Part model, mm, in its own coordinate system. A direction names the side the tool comes from. Coordinates: 2 decimals unless noted, no trailing zeros. Order: outer loops, then holes, each group sorted by start corner. A loop starts at its lowest first (then second) coordinate and runs counter-clockwise, first axis right, second up. Notation, with made-up numbers: M -12,-24.5 L 44,-24.5 A11 cw 44,-15.5 Z; hole C -37,83 d3. An arc over 180 degrees is marked long. Answer in a Markdown table with one row per item. Add a question column.
from build123d import *

# Parameters (mm, degrees)
SKETCH1_W             = 42
SKETCH1_H             = 42
BOSS_EXTRUDE1_DEPTH   = 36
SKETCH2_OUTSIDE_W     = 57.892
SKETCH2_OUTSIDE_H     = 57.892
SKETCH2_OUTSIDE_R     = 11
CUT_EXTRUDE1_DEPTH    = 2
FILLET1_R             = 0.5
SKETCH3_R             = 4
CUT_EXTRUDE2_DEPTH    = 3
SKETCH4_R             = 2.5
BOSS_EXTRUDE2_DEPTH   = 27
FILLET3_R             = 1
SKETCH5_R             = 12
BOSS_EXTRUDE3_DEPTH   = 0.5
FILLET4_R             = 0.1
M3_TAPPED_HOLE1_D     = 2.5
M3_TAPPED_HOLE1_DEPTH = 1
M3_TAPPED_HOLE1_TIP   = 0.751075774
CHAMFER2_SIZE         = 5
BOSS_EXTRUDE4_DEPTH   = 0.2
CUT_EXTRUDE4_START    = -10
CUT_EXTRUDE4_DEPTH    = 10
BOSS_EXTRUDE5_START   = -34.2
BOSS_EXTRUDE5_DEPTH   = 8
M3_TAPPED_HOLE3_D     = 2.5
M3_TAPPED_HOLE3_DEPTH = 1
M3_TAPPED_HOLE3_TIP   = 0.751075774


with BuildPart() as part:
    # Sketch1 → Boss-Extrude1 (new body)
    with BuildSketch(Plane.XY):
        Rectangle(SKETCH1_W, SKETCH1_H)
    extrude(amount=BOSS_EXTRUDE1_DEPTH)

    # Sketch2 outside → Cut-Extrude1 (cut)
    with BuildSketch(Plane.XY.offset(36)):
        Rectangle(SKETCH2_OUTSIDE_W, SKETCH2_OUTSIDE_H)
        Circle(SKETCH2_OUTSIDE_R, mode=Mode.SUBTRACT)
    extrude(amount=-CUT_EXTRUDE1_DEPTH, mode=Mode.SUBTRACT)

    # Fillet1
    fillet1_edges = [part.edges().sort_by_distance(p)[0] for p in [
        (-11, 0, 36),
    ]]
    fillet(fillet1_edges, radius=FILLET1_R)

    # Sketch3 → Cut-Extrude2 (cut)
    with BuildSketch(Plane.XY.offset(36)):
        Circle(SKETCH3_R)
    extrude(amount=-CUT_EXTRUDE2_DEPTH, mode=Mode.SUBTRACT)

    # Sketch4 → Boss-Extrude2 (add)
    with BuildSketch(Plane.XY.offset(33)):
        Circle(SKETCH4_R)
    extrude(amount=BOSS_EXTRUDE2_DEPTH)

    # Fillet3
    fillet3_edges = [part.edges().sort_by_distance(p)[0] for p in [
        (-2.5, 0, 60),
    ]]
    fillet(fillet3_edges, radius=FILLET3_R)

    # Sketch5 → Boss-Extrude3 (add)
    with BuildSketch(Plane.XY.offset(34)):
        Circle(SKETCH5_R)
    extrude(amount=BOSS_EXTRUDE3_DEPTH)

    # Fillet4
    fillet4_edges = [part.edges().sort_by_distance(p)[0] for p in [
        (-11, 0, 34.5),
    ]]
    fillet(fillet4_edges, radius=FILLET4_R)

    # M3 Tapped Hole1
    with Locations(Plane.XY.offset(34)):
        with Locations((15.5, 15.5), (-15.5, 15.5), (15.5, -15.5), (-15.5, -15.5)):
            Hole(M3_TAPPED_HOLE1_D / 2, depth=M3_TAPPED_HOLE1_DEPTH)
            with Locations((0, 0, -(M3_TAPPED_HOLE1_DEPTH + M3_TAPPED_HOLE1_TIP / 2))):  # 118° drill point
                Cone(0, M3_TAPPED_HOLE1_D / 2, M3_TAPPED_HOLE1_TIP, mode=Mode.SUBTRACT)

    # Chamfer2
    chamfer2_edges = [part.edges().sort_by_distance(p)[0] for p in [
        (21, -21, 17),
        (-21, -21, 17),
        (-21, 21, 17),
        (21, 21, 17),
    ]]
    chamfer(chamfer2_edges, length=CHAMFER2_SIZE)

    # Sketch9 → Boss-Extrude4 (add)
    with BuildSketch(Plane.XY.offset(34)):
        with BuildLine():
            Line((16, 21), (21, 16))
            Line((21, 16), (21, 10.138100447))
            Line((21, 10.138100447), (14.858342654, 10.138100447))
            ThreePointArc((14.858342654, 10.138100447), (11.322808748, 11.602566541), (9.858342654, 15.138100447))
            Line((9.858342654, 15.138100447), (9.858342654, 21))
            Line((9.858342654, 21), (16, 21))
        make_face()
        with BuildLine():
            Line((-21, 10.138100447), (-21, 16))
            Line((-21, 16), (-16, 21))
            Line((-16, 21), (-9.858342654, 21))
            Line((-9.858342654, 21), (-9.858342654, 15.138100447))
            ThreePointArc((-9.858342654, 15.138100447), (-11.322808748, 11.602566541), (-14.858342654, 10.138100447))
            Line((-14.858342654, 10.138100447), (-21, 10.138100447))
        make_face()
        with BuildLine():
            Line((-16, -21), (-21, -16))
            Line((-21, -16), (-21, -10.138100447))
            Line((-21, -10.138100447), (-14.858342654, -10.138100447))
            ThreePointArc((-14.858342654, -10.138100447), (-11.322808748, -11.602566541), (-9.858342654, -15.138100447))
            Line((-9.858342654, -15.138100447), (-9.858342654, -21))
            Line((-9.858342654, -21), (-16, -21))
        make_face()
        with BuildLine():
            Line((21, -10.138100447), (21, -16))
            Line((21, -16), (16, -21))
            Line((16, -21), (9.858342654, -21))
            Line((9.858342654, -21), (9.858342654, -15.138100447))
            ThreePointArc((9.858342654, -15.138100447), (11.322808748, -11.602566541), (14.858342654, -10.138100447))
            Line((14.858342654, -10.138100447), (21, -10.138100447))
        make_face()
    extrude(amount=BOSS_EXTRUDE4_DEPTH)

    # Sketch10 → Cut-Extrude4 (cut)
    with BuildSketch(Plane.XY.offset(34).offset(CUT_EXTRUDE4_START)):
        Polygon((21, 16.017915508), (16.017915508, 21), (-15.980285858, 21.03762965), (-21, 16.017915508), (-21, -16.050170564), (-16.050170564, -21), (16.010758898, -21), (21, -16.010758898), align=None)
        Polygon((19, -14), (14, -19), (-14, -19), (-19, -14), (-19, 14), (-14, 19), (14, 19), (19, 14), align=None, mode=Mode.SUBTRACT)
    extrude(amount=-CUT_EXTRUDE4_DEPTH, mode=Mode.SUBTRACT)

    # Sketch13 → Boss-Extrude5 (add)
    with BuildSketch(Plane.XY.offset(34.2).offset(BOSS_EXTRUDE5_START)):
        Polygon((-12.5, -25.6), (12.5, -25.6), (12.5, -23.3), (13.7, -23.3), (16, -21), (12.5, -21), (-12.5, -21), (-16, -21), (-13.7, -23.3), (-12.5, -23.3), align=None)
    extrude(amount=BOSS_EXTRUDE5_DEPTH)

    # M3 Tapped Hole3
    with Locations(Plane.XY.offset(34.2)):
        with Locations((-15.5, 15.5), (15.5, 15.5), (15.5, -15.5), (-15.5, -15.5)):
            Hole(M3_TAPPED_HOLE3_D / 2, depth=M3_TAPPED_HOLE3_DEPTH)
            with Locations((0, 0, -(M3_TAPPED_HOLE3_DEPTH + M3_TAPPED_HOLE3_TIP / 2))):  # 118° drill point
                Cone(0, M3_TAPPED_HOLE3_D / 2, M3_TAPPED_HOLE3_TIP, mode=Mode.SUBTRACT)


solid = part.part
(1) Slice it at B-B (y = -18). List the corners of the cut face in (x, z).
(2) Wall check: line 1 (Y direction, x = -15.5, z = 33.4); line 2 (Z direction, x = -3, y = -2). Give the ranges that are in metal, low to high.
(3) 3-axis set-ups, long thin cutter, end or side, ignore diameter. For faces 4 (the flat face through (-14, -15, 34.2)), 5 (the flat face through (2, 2, 33)), 6 (the flat face through (0, 19, 19)): which of +Z, -Z, +X, -X, +Y, -Y reach the whole face in a straight line?
(4) Pull direction X, two halves, no side cores. Call faces 1 (the conical face through (15.45, 15.29, 32.38)), 2 (the flat face through (-19, 0, 19)), 3 (the flat face through (0, -23, 8)): pulls with the +X half, pulls with the -X half, needs draft (parallel to the pull), parting line crosses it, or undercut.
(5) Drop flat-ended pins along their axis: P1, Ø12.5, axis at x = 5.5, y = 4, coming from the -Z side; P2, Ø1.3, axis at x = -13.5, z = 3.5, coming from the -Y side; P3, Ø2, axis at x = -8.5, y = -14.5, coming from the +Z side; P4, Ø8.5, axis at x = 16, y = 13.5, coming from the +Z side. Give the stop position or say it passes through.
(6) Slice it at C-C (z = 53). List the corners of the cut face in (x, y).
(7) Slice it at A-A (z = 30.5). List the corners of the cut face in (x, y), and give its area (3 significant figures).
Computed:
| question | item | result |
|---|---|---|
| 1 | outline | M -19,0 L 19,0 L 19,14 L 15,14 L 15,24 L 19,24 L 19,34.2 L 9.86,34.2 L 9.86,34 L -9.86,34 L -9.86,34.2 L -19,34.2 L -19,24 L -15,24 L -15,14 L -19,14 Z |
| 2 | line 1 | y = -21 to -16.75, -14.25 to 14.25, 16.75 to 21 |
| 2 | line 2 | z = 0 to 33, 34 to 34.5 |
| 3 | face 4 | +Z, -X, -Y |
| 3 | face 5 | none |
| 3 | face 6 | +X, -X, +Y |
| 4 | face 1 | undercut |
| 4 | face 2 | pulls with the -X half |
| 4 | face 3 | needs draft |
| 5 | P1 | stops at z = 0 |
| 5 | P2 | stops at y = -23.3 |
| 5 | P3 | stops at z = 34 |
| 5 | P4 | stops at z = 34.2 |
| 6 | outline | C 0,0 d5 |
| 7 | outline | M -21,-16 L -16,-21 L 16,-21 L 21,-16 L 21,16 L 16,21 L -16,21 L -21,16 Z |
| 7 | area | 1,710 mm^2 |
